```python
from build123d import *

# Parameters (mm, degrees)
SKETCH_1_R          = 0.6
SKETCH_1_W          = 24
SKETCH_1_H          = 12.5
EXTRUDE_1_DEPTH     = 1.45
CUT_EXTRUDE_1_DEPTH = 3
FILLET_1_R          = 0.5


with BuildPart() as part:
    # 草图1 → 凸台-拉伸1 (new body, symmetric)
    with BuildSketch(Plane.XY):
        with BuildLine():
            Line((-75, 12.6), (75, 12.6))
            ThreePointArc((75, 12.6), (87.6, 0), (75, -12.6))
            Line((75, -12.6), (-75, -12.6))
            ThreePointArc((-75, -12.6), (-87.6, 0), (-75, 12.6))
        make_face()
        with Locations((-43.55, 0)):
            Circle(SKETCH_1_R, mode=Mode.SUBTRACT)
        with Locations((-70.95, 0)):
            Circle(SKETCH_1_R, mode=Mode.SUBTRACT)
        with Locations((70.95, 0)):
            Circle(SKETCH_1_R, mode=Mode.SUBTRACT)
        with Locations((43.55, 0)):
            Circle(SKETCH_1_R, mode=Mode.SUBTRACT)
        with Locations((-57.25, 0)):
            Rectangle(SKETCH_1_W, SKETCH_1_H, mode=Mode.SUBTRACT)
        with Locations((57.25, 0)):
            Rectangle(SKETCH_1_W, SKETCH_1_H, mode=Mode.SUBTRACT)
    extrude(amount=EXTRUDE_1_DEPTH, both=True)

    # 草图2 → 切除-拉伸1 (cut)
    with BuildSketch(Plane.XY.offset(1.45)):
        with BuildLine():
            Line((44.45, 6.25), (44.05, 6.25))
            ThreePointArc((44.05, 6.25), (43.484314575, 6.015685425), (43.25, 5.45))
            Line((43.25, 5.45), (43.25, 3.85))
            ThreePointArc((43.25, 3.85), (43.484314575, 3.284314575), (44.05, 3.05))
            Line((44.05, 3.05), (45.25, 3.05))
            Line((45.25, 3.05), (45.25, 6.25))
            Line((45.25, 6.25), (69.25, 6.25))
            Line((69.25, 6.25), (69.25, 3.05))
            Line((69.25, 3.05), (70.45, 3.05))
            ThreePointArc((70.45, 3.05), (71.015685425, 3.284314575), (71.25, 3.85))
            Line((71.25, 3.85), (71.25, 5.45))
            ThreePointArc((71.25, 5.45), (71.015685425, 6.015685425), (70.45, 6.25))
            Line((70.45, 6.25), (70.05, 6.25))
            ThreePointArc((70.05, 6.25), (69.484314575, 6.484314575), (69.25, 7.05))
            Line((69.25, 7.05), (69.25, 9.15))
            Line((69.25, 9.15), (45.25, 9.15))
            Line((45.25, 9.15), (45.25, 7.05))
            ThreePointArc((45.25, 7.05), (45.015685425, 6.484314575), (44.45, 6.25))
        make_face()
        with BuildLine():
            Line((44.05, -3.05), (45.25, -3.05))
            Line((45.25, -3.05), (45.25, -6.25))
            Line((45.25, -6.25), (69.25, -6.25))
            Line((69.25, -6.25), (69.25, -3.05))
            Line((69.25, -3.05), (70.45, -3.05))
            ThreePointArc((70.45, -3.05), (71.015685425, -3.284314575), (71.25, -3.85))
            Line((71.25, -3.85), (71.25, -5.45))
            ThreePointArc((71.25, -5.45), (71.015685425, -6.015685425), (70.45, -6.25))
            Line((70.45, -6.25), (70.05, -6.25))
            ThreePointArc((70.05, -6.25), (69.484314575, -6.484314575), (69.25, -7.05))
            Line((69.25, -7.05), (69.25, -9.15))
            Line((69.25, -9.15), (45.25, -9.15))
            Line((45.25, -9.15), (45.25, -7.05))
            ThreePointArc((45.25, -7.05), (45.015685425, -6.484314575), (44.45, -6.25))
            Line((44.45, -6.25), (44.05, -6.25))
            ThreePointArc((44.05, -6.25), (43.484314575, -6.015685425), (43.25, -5.45))
            Line((43.25, -5.45), (43.25, -3.85))
            ThreePointArc((43.25, -3.85), (43.484314575, -3.284314575), (44.05, -3.05))
        make_face()
        with BuildLine():
            Line((-45.25, 3.05), (-45.25, 6.25))
            Line((-45.25, 6.25), (-69.25, 6.25))
            Line((-69.25, 6.25), (-69.25, 3.05))
            Line((-69.25, 3.05), (-70.45, 3.05))
            ThreePointArc((-70.45, 3.05), (-71.015685425, 3.284314575), (-71.25, 3.85))
            Line((-71.25, 3.85), (-71.25, 5.45))
            ThreePointArc((-71.25, 5.45), (-71.015685425, 6.015685425), (-70.45, 6.25))
            Line((-70.45, 6.25), (-70.05, 6.25))
            ThreePointArc((-70.05, 6.25), (-69.484314575, 6.484314575), (-69.25, 7.05))
            Line((-69.25, 7.05), (-69.25, 9.15))
            Line((-69.25, 9.15), (-45.25, 9.15))
            Line((-45.25, 9.15), (-45.25, 7.05))
            ThreePointArc((-45.25, 7.05), (-45.015685425, 6.484314575), (-44.45, 6.25))
            Line((-44.45, 6.25), (-44.05, 6.25))
            ThreePointArc((-44.05, 6.25), (-43.484314575, 6.015685425), (-43.25, 5.45))
            Line((-43.25, 5.45), (-43.25, 3.85))
            ThreePointArc((-43.25, 3.85), (-43.484314575, 3.284314575), (-44.05, 3.05))
            Line((-44.05, 3.05), (-45.25, 3.05))
        make_face()
        with BuildLine():
            Line((-45.25, -7.05), (-45.25, -9.15))
            Line((-45.25, -9.15), (-69.25, -9.15))
            Line((-69.25, -9.15), (-69.25, -7.05))
            ThreePointArc((-69.25, -7.05), (-69.484314575, -6.484314575), (-70.05, -6.25))
            Line((-70.05, -6.25), (-70.45, -6.25))
            ThreePointArc((-70.45, -6.25), (-71.015685425, -6.015685425), (-71.25, -5.45))
            Line((-71.25, -5.45), (-71.25, -3.85))
            ThreePointArc((-71.25, -3.85), (-71.015685425, -3.284314575), (-70.45, -3.05))
            Line((-70.45, -3.05), (-69.25, -3.05))
            Line((-69.25, -3.05), (-69.25, -6.25))
            Line((-69.25, -6.25), (-45.25, -6.25))
            Line((-45.25, -6.25), (-45.25, -3.05))
            Line((-45.25, -3.05), (-44.05, -3.05))
            ThreePointArc((-44.05, -3.05), (-43.484314575, -3.284314575), (-43.25, -3.85))
            Line((-43.25, -3.85), (-43.25, -5.45))
            ThreePointArc((-43.25, -5.45), (-43.484314575, -6.015685425), (-44.05, -6.25))
            Line((-44.05, -6.25), (-44.45, -6.25))
            ThreePointArc((-44.45, -6.25), (-45.015685425, -6.484314575), (-45.25, -7.05))
        make_face()
    extrude(amount=-CUT_EXTRUDE_1_DEPTH, mode=Mode.SUBTRACT)

    # 圆角1
    fillet_1_edges = [part.edges().sort_by_distance(p)[0] for p in [
        (69.25, -3.05, 0),
        (-69.25, 3.05, 0),
        (45.25, -3.05, 0),
        (-45.25, 3.05, 0),
        (-45.25, -3.05, 0),
        (-69.25, -3.05, 0),
        (69.25, 3.05, 0),
        (45.25, 3.05, 0),
    ]]
    fillet(fillet_1_edges, radius=FILLET_1_R)


solid = part.part
```
Geometry: final body of the model. Coordinates: model frame, mm. A direction names the side the tool comes from. Round coordinates to 2 decimals unless told otherwise and drop trailing zeros. Write each loop counter-clockwise with the first axis right and the second up, starting at its lowest first coordinate (ties: lowest second). Pieces come first, ordered by that corner, then holes. Notation, with made-up numbers: M 39,55.25 L 97,55.25 A19 cw 97,70.25 Z; hole C 71.25,19.25 d9. An arc over 180 degrees is marked long. Answer in a Markdown table with one row per item. Add a question column.
(1) Ray query, L1, parallel to X at y = -5, z = 0.75; L2, parallel to Y at x = -43.55, z = 0.35; L3, parallel to X at y = 5.5, z = 0.6. Return the intervals inside material, ascending.
(2) Contact query for flat-ended pins moving along their axis: pin 1 (0.6 mm diameter, centred on y = 8.5, z = 0.5, fed in from +X); pin 2 (1.1 mm diameter, centred on y = 7.5, z = 0, fed in from +X). Output: stop coordinate, or through.
(3) Cut plane B-B, the plane y = 11. Return the cut outline in (x, z), then the cut area to 3 significant figures.
(4) Draft query along Y for faces 1 (the face through (69.25, 0, 0)), 2 (the face through (1, 0, 1.45)), 3 (the face through (1, -12.6, 0)), 4 (the face through (87.597, 0.277, 0.02)). Return one class per face: pulls with the +Y half, pulls with the -Y half, needs draft (parallel to the pull), parting line crosses it, or undercut.
(5) Cut plane A-A, the plane z = 0.65. Give the number of separate pieces and of enclosed holes in the cut face, then the cut area to 3 significant figures.
(6) Reachability of faces 5 (the face through (-1, 12.6, 0)), 6 (the face through (57, 9.15, 0)) from +Z, -Z, +X, -X, +Y, -Y: full face, straight path, thin tool, end or side. Return the list, or none.
Established:
| question | item | result |
|---|---|---|
| 1 | L1 | -86.57 to -71.25, -43.25 to 43.25, 71.25 to 86.57 |
| 1 | L2 | -12.6 to -6.07, -3.23 to -0.6, 0.6 to 3.23, 6.07 to 12.6 |
| 1 | L3 | -86.34 to -71.25, -43.25 to 43.25, 71.25 to 86.34 |
| 2 | pin 1 | x = 84.57 |
| 2 | pin 2 | x = 85.51 |
| 3 | outline | M -81.14,-1.45 L 81.14,-1.45 L 81.14,1.45 L -81.14,1.45 Z |
| 3 | area | 471 mm² |
| 4 | face 1 | undercut |
| 4 | face 2 | needs draft |
| 4 | face 3 | pulls with the -Y half |
| 4 | face 4 | parting line crosses it |
| 5 | separate pieces | 1 |
| 5 | enclosed holes | 6 |
| 5 | area | 3,350 mm² |
| 6 | face 5 | +Z, -Z, +X, -X, +Y |
| 6 | face 6 | +Z, -Z |
